Design review of the part shown in the three views and the two pictorial views. Dimensions are in mm from the part's minimum x, y and z. A direction names the side the tool comes from. Coordinates: 2 decimals unless noted, no trailing zeros. One line per item, written item: value. Start each with the question number.
1. For the marked faces 1 and 2, list the 3-axis set-ups (+Z, -Z, +X, -X, +Y, -Y) from which the entire face can be reached by the end or side of a thin tool; tool diameter is ignored.
2. To check wall thickness, follow line 1 (Y direction, x = 9.5, z = 3.5); line 2 (X direction, y = 7.5, z = 2); line 3 (Z direction, x = 1.25, y = 12) (1 decimal). State the ranges of each line that lie inside material, in increasing order. Write a range as from..to.
3. The part is to be moulded in two halves that separate along Y. For the marked faces 3, 4 and 5, say which applies: released by +Y, released by -Y, zero draft, split by the parting line, or undercut.
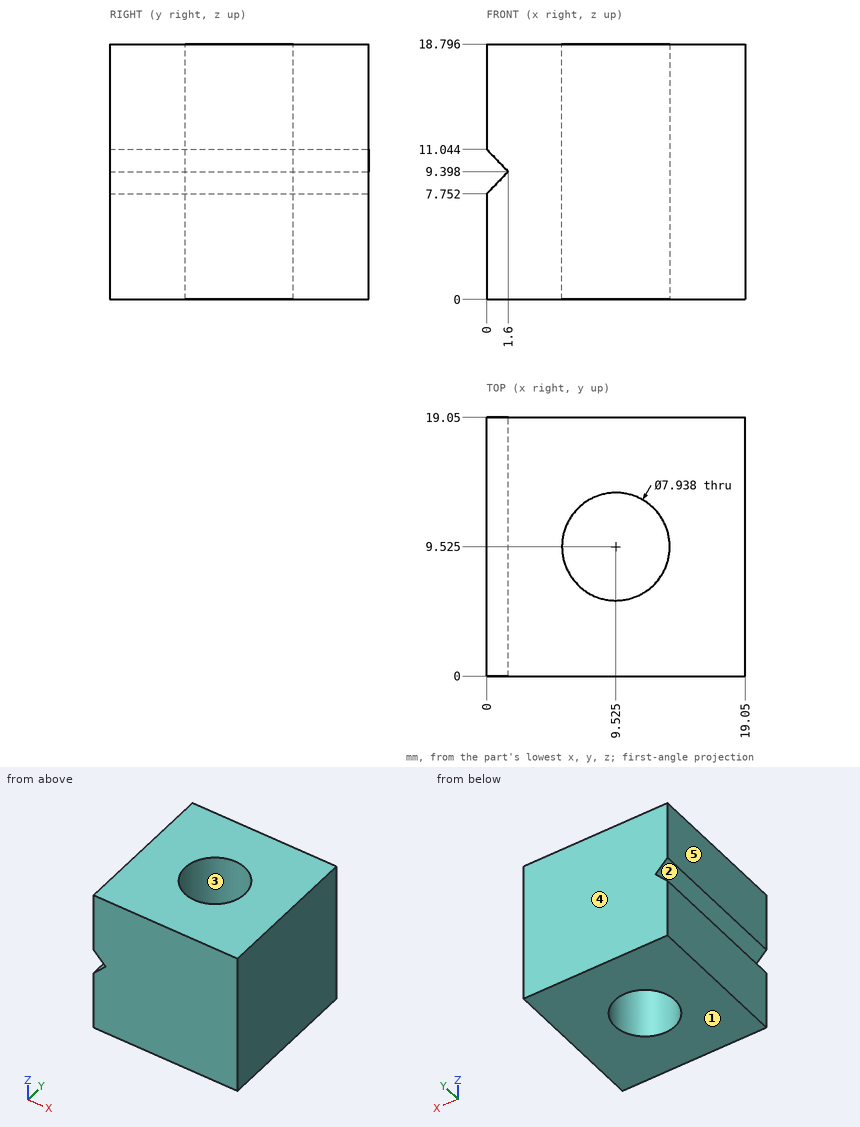
Solutions:
1. face 1: -Z, +X, -X, +Y, -Y
1. face 2: -X, +Y, -Y
2. line 1: 0..5.56, 13.49..19.05
2. line 2: 0..6.11, 12.94..19.05
2. line 3: 0..9, 9.8..18.8
3. face 3: undercut
3. face 4: released by +Y
3. face 5: zero draft
